from build123d import *

# Parameters (mm, degrees)
SKETCH1_W           = 25
SKETCH1_H           = 27
BOSS_EXTRUDE1_DEPTH = 12
CUT_EXTRUDE1_DEPTH  = 9
CUT_EXTRUDE2_DEPTH  = 26
FILLET1_R           = 16
CHAMFER2_SIZE       = 1
CHAMFER2_SIZE2      = 2
CHAMFER3_SIZE       = 1
CHAMFER3_SIZE2      = 2
CUT_EXTRUDE4_DEPTH  = 12
FILLET2_R           = 2
SKETCH6_R           = 4
CUT_EXTRUDE5_DEPTH  = 10


with BuildPart() as part:
    # Sketch1 → Boss-Extrude1 (new body)
    with BuildSketch(Plane.XY):
        with Locations((-12.5, 7.5)):
            Rectangle(SKETCH1_W, SKETCH1_H)
    extrude(amount=BOSS_EXTRUDE1_DEPTH)

    # Sketch2 → Cut-Extrude1 (cut)
    with BuildSketch(Plane.XY.offset(12)):
        with BuildLine():
            Line((0, 0), (-25, 0))
            Line((-25, 0), (-25, 2))
            Line((-25, 2), (-21, 2))
            ThreePointArc((-21, 2), (-15, 8), (-9, 2))
            Line((-9, 2), (0, 2))
            Line((0, 2), (0, 0))
        make_face()
        Polygon((0, 12), (-12, 12), (-12, 13.5), (-9.096, 13.5), (-8.596, 13), (-8.096, 13), (-7.596, 13.5), (-7.064, 13.5), (-6.564, 13), (-6.064, 13), (-5.564, 13.5), (-5.032, 13.5), (-4.532, 13), (-4.032, 13), (-3.532, 13.5), (-3, 13.5), (-2.5, 13), (-2, 13), (-1.5, 13.5), (0, 13.5), align=None)
    extrude(amount=-CUT_EXTRUDE1_DEPTH, mode=Mode.SUBTRACT)

    # Sketch3 → Cut-Extrude2 (cut, through all)
    with BuildSketch(Plane(origin=(0, 0, 0), x_dir=(0, 0, -1), z_dir=(1, 0, 0))):
        with BuildLine():
            Line((-6.5, -5.1), (-14.907534026, -5.1))
            Line((-14.907534026, -5.1), (-14.907534026, -15))
            Line((-14.907534026, -15), (-6.5, -15))
            ThreePointArc((-6.5, -15), (-1.55, -10.05), (-6.5, -5.1))
        make_face()
    extrude(amount=-CUT_EXTRUDE2_DEPTH, mode=Mode.SUBTRACT)

    # Fillet1
    fillet1_edges = [part.edges().sort_by_distance(p)[0] for p in [
        (-25, 21, 6),
    ]]
    fillet(fillet1_edges, radius=FILLET1_R)

    # Chamfer2
    chamfer2_edges = [part.edges().sort_by_distance(p)[0] for p in [
        (-4.5, 2, 12),
        (-23, 2, 12),
    ]]
    chamfer2_side = [part.faces().sort_by_distance(p)[0] for p in [
        (-10.97729814, 11.640214696, 12),
    ]]
    chamfer(chamfer2_edges, length=CHAMFER2_SIZE, length2=CHAMFER2_SIZE2, reference=chamfer2_side[0])

    # Chamfer3
    chamfer3_edges = [part.edges().sort_by_distance(p)[0] for p in [
        (-12.5, 0, 12),
    ]]
    chamfer3_side = [part.faces().sort_by_distance(p)[0] for p in [
        (-12.5, -2.55, 12),
    ]]
    chamfer(chamfer3_edges, length=CHAMFER3_SIZE, length2=CHAMFER3_SIZE2, reference=chamfer3_side[0])

    # Sketch5 → Cut-Extrude4 (cut)
    with BuildSketch(Plane(origin=(0, 0, 0), x_dir=(0, 0, -1), z_dir=(1, 0, 0))):
        Polygon((-12, 14.5), (-8.5, 12.75), (-12, 11), (-12, 12), (-12, 13.5), align=None)
    extrude(amount=-CUT_EXTRUDE4_DEPTH, mode=Mode.SUBTRACT)

    # Fillet2
    fillet2_edges = [part.edges().sort_by_distance(p)[0] for p in [
        (-9, 2, 6.5),
        (-21, 2, 6.5),
    ]]
    fillet(fillet2_edges, radius=FILLET2_R)

    # Sketch6 → Cut-Extrude5 (cut)
    with BuildSketch(Plane.XY.offset(12)):
        with Locations((-15, 0.794645258)):
            Circle(SKETCH6_R)
    extrude(amount=-CUT_EXTRUDE5_DEPTH, mode=Mode.SUBTRACT)


solid = part.part
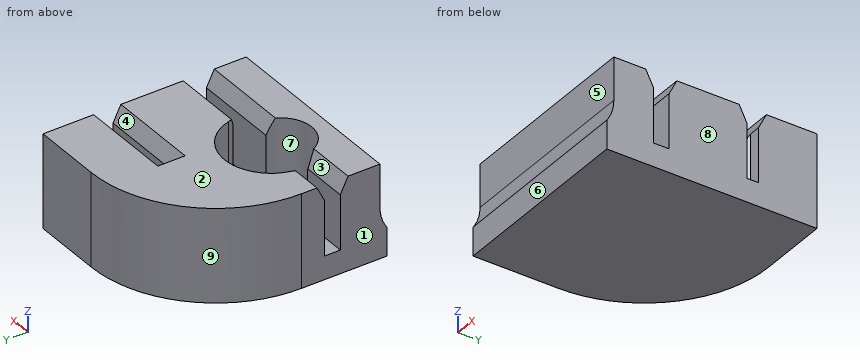
Can you work these out from the model? Positions are in its coordinate system, mm. Face numbers are marked on the shaded views. A direction names the side the tool comes from. Coordinates: 2 decimals unless noted, no trailing zeros. Loops run counter-clockwise (first coordinate to the right, second up) from the corner with the lowest first, then second, coordinate; pieces in that order, holes last. Notation, with made-up numbers: M -26,-25.5 L 29,-25.5 A20 cw 29,-9.5 Z; hole C -20,19.25 d2. An arc over 180 degrees is marked long. Answer as CSV lines item,"result". Start each with the question number.
1. For pin 1 Ø0.9 at (x, z) = (-11, 5) entering from -Y; pin 2 Ø3 at (x, z) = (-11, 9) entering from -Y; pin 3 Ø0.6 at (x, z) = (-5.5, 5) entering from -Y, each with a flat end and sliding along its axis, tell me the tip position at first contact or that it passes through.
2. If I drill on probe 1 along Y at (x, z) = (-1.5, 8); probe 2 along Y at (x, z) = (-10.25, 9.75); probe 3 along Z at (x, y) = (-14, 6.75), over which ranges is the centre line in solid material (lowest first)? Write a range as [from, to].
3. Thinking about a two-plate mould opening in X: for the marked faces 6, 7, 8 and 9, which applies, +X half, -X half, draft (parallel to the pull), parting line (faces both ways), or undercut?
4. For the marked faces 1, 2, 3, 4 and 5, which set-ups out of +Z, -Z, +X, -X, +Y, -Y let a thin tool reach every point of the face, with its end or its side?
5. Suppose I cut it at C-C, the plane y = 8.75. List the corners of the cut face in (x, z) for me.
6. Suppose I cut it at B-B, the plane y = 18. List the corners of the cut face in (x, z) for me.
7. Suppose I cut it at A-A, the plane x = -13.5. List the corners of the cut face in (y, z) for me.
Output:
1,pin 1,"stops at y = -5.5"
1,pin 2,"stops at y = -5.1"
1,pin 3,"stops at y = -5.44"
2,probe 1,"y = [-5.1, 0], [2, 12], [13.5, 21]"
2,probe 2,"y = [-5.1, 0], [5.67, 12], [13.5, 20.95]"
2,probe 3,"z = [0, 3]"
3,face 6,"draft"
3,face 7,"undercut"
3,face 8,"+X half"
3,face 9,"-X half"
4,face 1,"+Z, -Z, -X, +Y, -Y"
4,face 2,"+Z, +X, -X, +Y, -Y"
4,face 3,"+Z, +X, -X"
4,face 4,"+Z, +X"
4,face 5,"+Z, +X, -X, -Y"
5,outline,"M -24.55,0 L 0,0 L 0,12 L -24.55,12 Z"
6,outline,"M -18.33,0 L 0,0 L 0,12 L -18.33,12 Z"
7,outline,"M -6,0 L 20.35,0 L 20.35,12 L 7.81,12 L 7.81,3 L 4.5,3 L 4.5,2 L -2.91,2 L -2.91,12 L -5.1,12 L -5.1,6.5 A4.95 cw -6,3.65 Z"
